Check sheet for the modelled part. Datum: model origin and axes. Units: mm. A direction names the side the tool comes from. Round coordinates to 2 decimals unless told otherwise and drop trailing zeros. Write each loop counter-clockwise with the first axis right and the second up, starting at its lowest first coordinate (ties: lowest second). Pieces come first, ordered by that corner, then holes. Notation, with made-up numbers: M 34,48 L 90,48 A14 ccw 90,56 Z; hole C 25.25,78 d5. An arc over 180 degrees is marked long. Put each result on its own line as item: value.
```python
from build123d import *

# Parameters (mm, degrees)
SKETCH11_R          = 3.96875
SKETCH11_R_2        = 15.08125
SKETCH11_R_3        = 2
BOSS_EXTRUDE2_DEPTH = 5.08


with BuildPart() as part:
    # Sketch11 → Boss-Extrude2 (new body)
    with BuildSketch(Plane(origin=(0, 0, 0), x_dir=(1, 0, 0), z_dir=(0, 1, 0))):
        with BuildLine():
            Line((19.05, -173.758834345), (19.05, -72.598586407))
            ThreePointArc((19.05, -72.598586407), (19.041478453, -72.390699795), (19.015970989, -72.184208077))
            Line((19.015970989, -72.184208077), (6.891420221, 1.139540409))
            ThreePointArc((6.891420221, 1.139540409), (-0.132898533, 6.983735604), (-6.929785414, 0.876526736))
            Line((-6.929785414, 0.876526736), (-22.088986057, -118.971508934))
            Line((-22.088986057, -118.971508934), (-25.39598653, -177.728690609))
            ThreePointArc((-25.39598653, -177.728690609), (-25.398996434, -177.800028219), (-25.4, -177.871422245))
            Line((-25.4, -177.871422245), (-25.4, -228.6))
            ThreePointArc((-25.4, -228.6), (-22.745272537, -232.230626029), (-18.480606107, -230.801765114))
            Line((-18.480606107, -230.801765114), (16.71464631, -181.098051393))
            ThreePointArc((16.71464631, -181.098051393), (18.452086765, -177.609742801), (19.05, -173.758834345))
        make_face()
        with Locations(Location((0, 0, 0), (0, 0, 270))):
            Circle(SKETCH11_R, mode=Mode.SUBTRACT)
        with Locations(Location((0, -160.246508934, 0), (0, 0, 270))):
            Circle(SKETCH11_R_2, mode=Mode.SUBTRACT)
        with Locations(Location((-20.32, -225.425, 0), (0, 0, 270))):
            Circle(SKETCH11_R_3, mode=Mode.SUBTRACT)
        with Locations(Location((-20.32, -219.075, 0), (0, 0, 270))):
            Circle(SKETCH11_R_3, mode=Mode.SUBTRACT)
        with Locations(Location((-20.32, -212.725, 0), (0, 0, 270))):
            Circle(SKETCH11_R_3, mode=Mode.SUBTRACT)
        with Locations(Location((-20.32, -206.375, 0), (0, 0, 270))):
            Circle(SKETCH11_R_3, mode=Mode.SUBTRACT)
        with Locations(Location((0, -16.51, 0), (0, 0, 270))):
            Circle(SKETCH11_R_3, mode=Mode.SUBTRACT)
        with Locations(Location((14.605, -176.756508934, 0), (0, 0, 270))):
            Circle(SKETCH11_R_3, mode=Mode.SUBTRACT)
        with BuildLine():
            Line((11.940278596, -80.334093652), (-12.090624848, -107.18518059))
            ThreePointArc((-12.090624848, -107.18518059), (-15.037374992, -107.802243553), (-16.503240932, -105.172540118))
            Line((-16.503240932, -105.172540118), (-7.115464935, -30.953157513))
            ThreePointArc((-7.115464935, -30.953157513), (-5.014621207, -26.986469282), (-0.815660013, -25.4))
            Line((-0.815660013, -25.4), (-0.124902871, -25.4))
            ThreePointArc((-0.124902871, -25.4), (3.982665997, -26.907440966), (6.140024603, -30.714054174))
            Line((6.140024603, -30.714054174), (13.473470783, -75.063389134))
            ThreePointArc((13.473470783, -75.063389134), (13.305815609, -77.87296697), (11.940278596, -80.334093652))
        make_face(mode=Mode.SUBTRACT)
        with BuildLine():
            Line((13.97, -141.812492878), (13.97, -90.426050798))
            ThreePointArc((13.97, -90.426050798), (12.336685433, -88.053389523), (9.537305885, -88.732147321))
            Line((9.537305885, -88.732147321), (-15.843545445, -117.091607347))
            ThreePointArc((-15.843545445, -117.091607347), (-16.487420873, -118.917476564), (-15.657551613, -120.666673802))
            Line((-15.657551613, -120.666673802), (9.723299718, -143.693655856))
            ThreePointArc((9.723299718, -143.693655856), (12.458732541, -144.134842843), (13.97, -141.812492878))
        make_face(mode=Mode.SUBTRACT)
        with BuildLine():
            Line((-13.582521272, -126.836237527), (-2.809524218, -136.610125984))
            ThreePointArc((-2.809524218, -136.610125984), (-2.003545388, -138.86283126), (-3.426980373, -140.785879825))
            Line((-3.426980373, -140.785879825), (-15.060903725, -146.30851259))
            ThreePointArc((-15.060903725, -146.30851259), (-17.567328552, -146.121811397), (-18.686134382, -143.87119009))
            Line((-18.686134382, -143.87119009), (-17.825208084, -128.574668869))
            ThreePointArc((-17.825208084, -128.574668869), (-16.252271294, -126.367052616), (-13.582521272, -126.836237527))
        make_face(mode=Mode.SUBTRACT)
        with BuildLine():
            Line((6.282161105, -189.238159376), (-3.018903236, -202.373380963))
            ThreePointArc((-3.018903236, -202.373380963), (-6.220540057, -204.429171418), (-9.951861921, -203.684866462))
            Line((-9.951861921, -203.684866462), (-16.757100161, -199.219099788))
            ThreePointArc((-16.757100161, -199.219099788), (-18.440171631, -197.385216843), (-19.05, -194.971927471))
            Line((-19.05, -194.971927471), (-19.05, -183.748869713))
            ThreePointArc((-19.05, -183.748869713), (-17.268890157, -179.885746141), (-13.174518217, -178.731538875))
            Line((-13.174518217, -178.731538875), (2.931784364, -181.28514172))
            ThreePointArc((2.931784364, -181.28514172), (6.817844364, -184.330274157), (6.282161105, -189.238159376))
        make_face(mode=Mode.SUBTRACT)
        with BuildLine():
            Line((3.834506832, -6.35), (-3.834506832, -6.35))
            ThreePointArc((-3.834506832, -6.35), (-4.67429907, -6.667293856), (-5.094467816, -7.460631503))
            Line((-5.094467816, -7.460631503), (-5.415744418, -10.000631503))
            ThreePointArc((-5.415744418, -10.000631503), (-5.108489577, -10.999792239), (-4.155783434, -11.43))
            Line((-4.155783434, -11.43), (4.254512077, -11.43))
            ThreePointArc((4.254512077, -11.43), (5.223023884, -10.981513774), (5.507497571, -9.952810835))
            Line((5.507497571, -9.952810835), (5.087492326, -7.412810835))
            ThreePointArc((5.087492326, -7.412810835), (4.656020605, -6.651488193), (3.834506832, -6.35))
        make_face(mode=Mode.SUBTRACT)
    extrude(amount=-BOSS_EXTRUDE2_DEPTH)


solid = part.part
```
1. Cross-section at C-C (y = -1.15). Count the separate pieces of the cut face and the enclosed holes in it, then the cut area to 3 significant figures.
Computed values:
separate pieces: 1
enclosed holes: 13
area: 3,460 mm2
2. Access from +Z, -Z, +X, -X, +Y, -Y to the whole of each face (thin tool, end or side, straight path). Record for faces 5 (the cylindrical face through (-16.289, -2.504, 126.383)), 6 (the flat face through (-25.4, -3, 203)).
Computed values:
face 5: +Y, -Y
face 6: +Z, -Z, -X, +Y, -Y
3. Scan lines: probe 1 along X at (y, z) = (-3.4, 136); probe 2 along X at (y, z) = (-4.4, 105.5); probe 3 along Z at (x, y) = (4.5, -3.8). Record each from-to range of solid material in increasing order.
Computed values:
probe 1: x = -23.05 to -18.24, -3.48 to 1.24, 13.97 to 19.05
probe 2: x = -20.39 to -16.52, -10.58 to -5.47, 13.97 to 19.05
probe 3: z = -5.34 to 6.54, 11.41 to 27.4, 88.65 to 94.36, 138.95 to 145.85, 174.64 to 181.81, 191.75 to 198.35
4. Cross-section at B-B (z = 114.5). Enter the section's corners in (x, y).
Computed values:
outline: M -21.52,-5.08 L -13.52,-5.08 L -13.52,0 L -21.52,0 Z; M 13.97,-5.08 L 19.05,-5.08 L 19.05,0 L 13.97,0 Z
5. Depth check by flat-ended pin: pin 1 Ø1.5 at (x, y) = (-7.5, -1) entering from +Z; pin 2 Ø2.5 at (y, z) = (-2.5, 111.5) entering from -X; pin 3 Ø1.5 at (x, y) = (1.5, -3) entering from -Z. Enter the tip coordinate at first touch or a pass-through.
Computed values:
pin 1: stops at z = 216.35
pin 2: stops at x = -21.3
pin 3: stops at z = -6.94
6. Release check for a two-part mould opening along Z. For faces 1 (the flat face through (-8, 0, 130)), 2 (the flat face through (0.093, -2.504, 93.572)), 3 (the flat face through (-23.72, -2.5, 147.94)), 4 (the flat face through (13.97, -3, 116)) record: +Z half, -Z half, draft (parallel to the pull), parting line (faces both ways), or undercut.
Computed values:
face 1: draft
face 2: undercut
face 3: -Z half
face 4: undercut
7. Cross-section at A-A (z = 16.51). Enter the section's corners in (x, y).
Computed values:
outline: M -9.13,-5.08 L -2,-5.08 L -2,0 L -9.13,0 Z; M 2,-5.08 L 9.81,-5.08 L 9.81,0 L 2,0 Z
